Autodesk Inventor part; units mm, degrees
ref_plane "YZ Plane" through (0, 0, 0) normal (1, 0, 0) x (0, 1, 0)
ref_plane "XZ Plane" through (0, 0, 0) normal (0, 1, 0) x (-1, 0, 0)
ref_plane "XY Plane" through (0, 0, 0) normal (0, 0, 1) x (1, 0, 0)
sketch "Sketch1" plane through (0, 0, 0) normal (0, 0, 1) x (1, 0, 0)
  line L0 (22, -19) -> (22, 19)
  line L1 (-19, -22) -> (19, -22)
  line L2 (22.5, 22.5) -> (22.5, -22.5)
  line L3 (22.5, -22.5) -> (-22.5, -22.5)
  line L4 (-22.5, -22.5) -> (-22.5, 22.5)
  line L5 (-22.5, 22.5) -> (22.5, 22.5)
  line L6 (22.5, 22.5) -> (-22.5, -22.5) construction
  line L7 (22.5, -22.5) -> (-22.5, 22.5) construction
  point P0 (0, 0)
  dimension "d0" = 45
  dimension "d1" = 45
extrude "Extrusion1" add sketch "Sketch1" along normal blind 0.1
sketch "Sketch2" plane through (22.5, -22.5, 0) normal (1, 0, 0) x (0, 0, -1)
  line L0 (-0.1, 0) -> (-0.1, 45)
  line L1 (0, 0) -> (0, 45)
  line L2 (0, 45) -> (-0.1, 45)
  line L3 (-0.1, 0) -> (-0.1, 45)
  line L4 (0, 0) -> (-0.1, 0)
  line L5 (-0.1, 0) -> (9.9, 0)
  line L6 (9.9, 0) -> (9.9, 45)
  line L7 (9.9, 45) -> (-0.1, 45)
  line L8 (-0.1, 45) -> (-0.1, 0)
  point P0 (0, 22.5)
  dimension "d4" = 10
  dimension "d5" = 45
extrude "Extrusion2" add sketch "Sketch2" along normal blind 0.1
chamfer "Chamfer1" distance 1 angle 45 2 edges at (22.55, -22.5, -9.9) (22.55, 22.5, -9.9)
chamfer "Chamfer2" distance 1 angle 45 2 edges at (-22.5, 22.5, 0.05) (-22.5, -22.5, 0.05)
properties part number "tag"
Build history of the part. All positions in model axes, mm. Give positions to 0.01 mm unless a question says otherwise; leave off trailing zeros. Write each loop counter-clockwise with the first axis right and the second up, starting at its lowest first coordinate (ties: lowest second). Pieces come first, ordered by that corner, then holes. Notation, with made-up numbers: (57.5, 27) - (114.5, 27) arc R16 cw to (114.5, 31) - close; hole circle Ø10 at (35.5, 25). An arc over 180 degrees is marked (long way). Use one line per item in the form item = value. Start each with the question number.
1. Band-saw the part on B-B on z = -5.75. Write the cut outline in (x, y), plus the area to 3 significant figures.
2. Band-saw the part on C-C on x = -8. Write the cut outline in (y, z).
3. Drop flat-ended pins along their axis: pin 1 Ø1 at (y, z) = (10.5, -5.5) entering from -X; pin 2 Ø1.5 at (x, y) = (6, -15.5) entering from -Z. Give the stop position or say it passes through.
4. Band-saw the part on A-A on y = 2. Write the cut outline in (x, z).
Conclusion:
q1.outline = (22.5, -22.5) - (22.6, -22.5) - (22.6, 22.5) - (22.5, 22.5) - close
q1.area = 4.50 mm²
q2.outline = (-22.5, 0) - (22.5, 0) - (22.5, 0.1) - (-22.5, 0.1) - close
q3.pin_1 = 22.5
q3.pin_2 = 0
q4.outline = (-22.5, 0) - (22.5, 0) - (22.5, -9.9) - (22.6, -9.9) - (22.6, 0.1) - (-22.5, 0.1) - close
